```python
from build123d import *

# Parameters (mm, degrees)
SKETCH1_W           = 113
SKETCH1_H           = 55
BOSS_EXTRUDE1_DEPTH = 3
BOSS_EXTRUDE3_DEPTH = 113
SKETCH2_R           = 2.25
BOSS_EXTRUDE2_DEPTH = 5
SHELL1_START        = -50.038745387
SHELL1_DEPTH        = 108
SKETCH4_W           = 88
SKETCH4_H           = 40.5
CUT_EXTRUDE1_DEPTH  = 10
FILLET2_R           = 3.5
CUT_EXTRUDE2_REACH  = 98.336
SKETCH5_W           = 45
SKETCH5_H           = 7
FILLET3_R           = 3


# Read off the part's stored shape, not the designer's step: Shell1
with BuildPart() as part:
    # Sketch1 → Boss-Extrude1 (new body)
    with BuildSketch(Plane(origin=(0, 0, 0), x_dir=(1, 0, 0), z_dir=(0, 1, 0))):
        with Locations((3.961254613, 12.529520295)):
            Rectangle(SKETCH1_W, SKETCH1_H)
    extrude(amount=BOSS_EXTRUDE1_DEPTH)

    # Sketch3 → Boss-Extrude3 (add)
    with BuildSketch(Plane(origin=(60.461254613, 0, 0), x_dir=(0, 0, -1), z_dir=(1, 0, 0))):
        Polygon((-14.970479705, 0), (-14.970479705, -50.990195136), (40.029520295, 0), align=None)
    extrude(amount=-BOSS_EXTRUDE3_DEPTH)

    # Sketch2 → Boss-Extrude2 (add)
    with BuildSketch(Plane(origin=(0, 3, 0), x_dir=(1, 0, 0), z_dir=(0, 1, 0))):
        with Locations(Location((-46.038745387, 31.709520295, 0), (0, 0, 270))):
            Circle(SKETCH2_R)
        with Locations(Location((53.961254613, 31.629520295, 0), (0, 0, 270))):
            Circle(SKETCH2_R)
        with Locations(Location((53.961254613, 1.029520295, 0), (0, 0, 270))):
            Circle(SKETCH2_R)
        with Locations(Location((-46.038745387, 1.029520295, 0), (0, 0, 270))):
            Circle(SKETCH2_R)
    extrude(amount=BOSS_EXTRUDE2_DEPTH)

    # Shell1 outline → Shell1 (cut)
    with BuildSketch(Plane.YZ.offset(SHELL1_START)):
        Polygon((0.5, 12.470479705), (-48.672458993, 12.470479705), (-2.317736143, -37.529520295), (0.5, -37.529520295), align=None)
    extrude(amount=SHELL1_DEPTH, mode=Mode.SUBTRACT)

    # Sketch4 → Cut-Extrude1 (cut)
    with BuildSketch(Plane.XZ.offset(-0.5)):
        with Locations((3.961254613, -10.279520295)):
            Rectangle(SKETCH4_W, SKETCH4_H)
    extrude(amount=-CUT_EXTRUDE1_DEPTH, mode=Mode.SUBTRACT)

    # Fillet2
    fillet2_edges = [part.edges().sort_by_distance(p)[0] for p in [
        (-52.538745387, 1.5, -40.029520295),
        (60.461254613, 1.5, -40.029520295),
        (60.461254613, -23.995097568, 14.970479705),
        (-52.538745387, -23.995097568, 14.970479705),
    ]]
    fillet(fillet2_edges, radius=FILLET2_R)

    # Cut-Extrude2: up to this face of the body (flat: up to its plane)
    cut_extrude2_end = Plane(part.part.faces().sort_by_distance((3.961254613, 1.75, -30.529520295))[0])
    # Sketch5 → Cut-Extrude2 (cut, up to the picked face)
    with BuildSketch(Plane.XY.offset(14.970479705), mode=Mode.PRIVATE) as cut_extrude2_sk1:
        with Locations((26.461254613, -0.5)):
            Rectangle(SKETCH5_W, SKETCH5_H)
    cut_extrude2_tool1 = split(extrude(cut_extrude2_sk1.sketch, amount=-CUT_EXTRUDE2_REACH, mode=Mode.PRIVATE), bisect_by=cut_extrude2_end, keep=Keep.BOTH, mode=Mode.PRIVATE)
    add(cut_extrude2_tool1.solids().sort_by(Axis((26.461255, -0.5, 14.97048), (0, 0, -1)))[0], mode=Mode.SUBTRACT)

    # Fillet3
    fillet3_edges = [part.edges().sort_by_distance(p)[0] for p in [
        (48.961254613, -4, 13.720479705),
        (3.961254613, -4, 13.720479705),
    ]]
    fillet(fillet3_edges, radius=FILLET3_R)


solid = part.part
```
The listing builds one solid part. Answer for the finished solid, in the listing's coordinates (mm). A direction names the side the tool comes from. Round coordinates to 2 decimals unless told otherwise and drop trailing zeros. Write each loop counter-clockwise with the first axis right and the second up, starting at its lowest first coordinate (ties: lowest second). Pieces come first, ordered by that corner, then holes. Notation, with made-up numbers: (50, 84) -> (82, 84) arc R15 cw to (82, 93) -> close; hole circle Ø7 at (31, 77). An arc over 180 degrees is marked (long way). Answer as a JSON object with one key per item and string values. Group by question number.
Q1. Section D-D (x = -1.5) is taken. Write down the section's boundary in (y, z).
Q2. Determine the mould class of faces 1 (the face through (4.225, -50.165, 14.08)), 2 (the face through (-48.035, 5.465, 0.009)), 3 (the face through (3.961, 1, 13)) for opening direction Z: pulls with the +Z half, pulls with the -Z half, needs draft (parallel to the pull), parting line crosses it, or undercut.
Q3. Each of these flat-tipped pins is pushed along its axis until it touches: pin 1 Ø15 at (x, y) = (30, -15.5) entering from -Z; pin 2 Ø2 at (x, y) = (11.5, 1.5) entering from +Z; pin 3 Ø25 at (x, z) = (25.5, -20.5) entering from -Y. Where does it stop, or does it pass through?
Q4. Section A-A (x = 41.5) is taken. Write down the section's boundary in (y, z).
Q5. Which of the six approach directions +Z, -Z, +X, -X, +Y, -Y give full straight-line access (tool end or side, diameter ignored) to faces 4 (the face through (3, 3, -31)), 5 (the face through (-51.49, -24.37, 13.97)), 6 (the face through (-46, 8, -32)), 7 (the face through (4.86, -3.14, 13.7)), 8 (the face through (4, 2, -30.53))?
Q6. Section C-C (y = -19) is taken. Write down the section's boundary in (x, z).
Q7. Straight lines are drawn through the part: line 1 along X through (y, z) = (-6.5, 7); line 2 along Z through (x, y) = (-6, -37); line 3 along Y through (x, z) = (51, -9). For each, find the intervals that lie inside material, in ascending order.
Q8. Section B-B (z = -21) is taken. Write down the section's boundary in (x, y), plus the area to 3 significant figures.
Check values:
{
 "1": {"outline": "(-50.99, 14.97) -> (-48.67, 12.47) -> (0.5, 12.47) -> (0.5, 9.97) -> (3, 9.97) -> (3, 14.97) -> close; (-2.32, -37.53) -> (0, -40.03) -> (3, -40.03) -> (3, -30.53) -> (0.5, -30.53) -> (0.5, -37.53) -> close"},
 "2": {"face 1": "pulls with the -Z half", "face 2": "undercut", "face 3": "needs draft"},
 "3": {"pin 1": "z = 12.47", "pin 2": "z = -30.53", "pin 3": "y = 0.5"},
 "4": {"outline": "(-50.99, 14.97) -> (-48.67, 12.47) -> (-4, 12.47) -> (-4, 14.97) -> close; (-2.32, -37.53) -> (0, -40.03) -> (3, -40.03) -> (3, -30.53) -> (0.5, -30.53) -> (0.5, -37.53) -> close"},
 "5": {"face 4": "+Y", "face 5": "+Z, -X, +Y, -Y", "face 6": "+Z, -Z, +X, -X, +Y", "face 7": "+Z, +Y", "face 8": "+Y, -Y"},
 "6": {"outline": "(-52.54, -19.54) -> (-50.04, -19.54) -> (-50.04, 12.47) -> (57.96, 12.47) -> (57.96, -19.54) -> (60.46, -19.54) -> (60.46, 11.47) arc R3.5 ccw to (56.96, 14.97) -> (-49.04, 14.97) arc R3.5 ccw to (-52.54, 11.47) -> close"},
 "7": {"line 1": "-52.54 to -50.04, 57.96 to 60.46", "line 2": "12.47 to 14.97", "line 3": "0.5 to 3"},
 "8": {"outline": "(-52.54, -17.64) -> (-50.04, -17.64) -> (-50.04, 0.5) -> (-40.04, 0.5) -> (-40.04, 3) -> (-52.54, 3) -> close; (48.96, 0.5) -> (57.96, 0.5) -> (57.96, -17.64) -> (60.46, -17.64) -> (60.46, 3) -> (48.96, 3) -> close", "area": "151 mm^2"}
}
